Autodesk Inventor part; units mm, degrees
ref_plane "YZ Plane" through (0, 0, 0) normal (1, 0, 0) x (0, 1, 0)
ref_plane "XZ Plane" through (0, 0, 0) normal (0, 1, 0) x (-1, 0, 0)
ref_plane "XY Plane" through (0, 0, 0) normal (0, 0, 1) x (1, 0, 0)
sketch "Sketch1" plane through (0, 0, 0) normal (0, 0, 1) x (1, 0, 0)
  circle A0 centre (0, 0) radius 37.465
  dimension "d0" = 74.93
extrude "Extrusion1" add sketch "Sketch1" along normal blind 2.54
sketch "Sketch3" plane through (0, 0, 0) normal (0, 0, -1) x (-1, 0, 0)
  circle A0 centre (0, 0) radius 4.191
  circle A1 centre (0, 0) radius 7.9375
  circle A2 centre (0, 0) radius 2.3813
  dimension "d4" = 8.382
  dimension "d5" = 15.875
  dimension "d6" = 4.7625
extrude "Extrusion3" cut sketch "Sketch3" against normal through all contours A0 | A2
extrude "Extrusion4" add sketch "Sketch3" along normal blind 5.08 contours A1
sketch "Sketch4" plane through (0, 0, 2.54) normal (0, 0, 1) x (1, 0, 0)
  line L0 (0, 0) -> (0, 30.48)
  circle A0 centre (0, 30.48) radius 1.905
  circle A1 centre (-26.3965, 15.24) radius 1.905
  circle A2 centre (-26.3965, -15.24) radius 1.905
  circle A3 centre (0, -30.48) radius 1.905
  circle A4 centre (26.3965, -15.24) radius 1.905
  circle A5 centre (26.3965, 15.24) radius 1.905
  dimension "d13" = 30.48
  dimension "d14" = 3.81
  dimension "d17" = 360
extrude "Extrusion5" cut sketch "Sketch4" against normal blind 25.4
sketch "Sketch6" plane through (0, 0, 2.54) normal (0, 0, 1) x (1, 0, 0)
  circle A0 centre (0, 0) radius 3.556
  circle A1 centre (0, 0) radius 4.191
  dimension "d21" = 7.112
extrude "Extrusion6" add sketch "Sketch6" against normal blind 1.27
chamfer "Chamfer1" distance 1.27 angle 45 6 edges at (-28.3015, -15.24, 2.54) (-28.3015, 15.24, 2.54) (-1.905, 30.48, 2.54) (-1.905, -30.48, 2.54) (24.4915, -15.24, 2.54) (24.4915, 15.24, 2.54)
sketch "Sketch7" plane through (0, 0, 2.54) normal (0, 0, 1) x (1, 0, 0)
  circle A0 centre (0, 19.05) radius 3.175
  point P0 (0, 0)
  dimension "d27" = 6.35
  dimension "d28" = 19.05
extrude "Extrusion7" cut sketch "Sketch7" against normal through all
fillet "Fillet1" radius 1.27 1 edges at (7.9375, 0, 0)
properties part number "SpoolEndFrontSide"
Model file for the job. Use its own axes, mm. A direction names the side the tool comes from. Give positions to 0.01 mm unless a question says otherwise; leave off trailing zeros. Order: outer loops, then holes, each group sorted by start corner. A loop starts at its lowest first (then second) coordinate and runs counter-clockwise, first axis right, second up.
1) Saw through at B-B, the plane y = -15.24. Write the cut outline in (x, z).
2) Saw through at A-A, the plane x = 0. Count the separate pieces of the cut face and the enclosed holes in it, then the cut area to 3 significant figures.
3) Wall check: probe 1 along Y at (x, z) = (0, 1.7) (3 decimals); probe 2 along Z at (x, y) = (-23, -6.5); probe 3 along Y at (x, z) = (-23, 2). Give the ranges that are in metal, low to high.
4) Mould opens along Y. For faces 3 (the cylindrical face through (-26.81, 13.38, 0.64)), 4 (the flat face through (8, -8, 0)), 5 (the cylindrical face through (-29.73, 22.8, 1.25)), 6 (the cylindrical face through (-0.69, 15.95, 1.29)) say: +Y half, -Y half, draft (parallel to the pull), parting line (faces both ways), or undercut.
5) 3-axis set-ups, long thin cutter, end or side, ignore diameter. For faces 1 (the cylindrical face through (-3.997, -1.259, -1.861)), 2 (the cylindrical face through (25.98, 13.38, 0.64)): which of +Z, -Z, +X, -X, +Y, -Y reach the whole face in a straight line?
6) Saw through at D-D, the plane z = -3.25. Write the cut outline in (x, y) (1 decimal), then the cut area to 3 significant figures.
7) Saw through at C-C, the plane y = 30.48. Write the cut outline in (x, z) (3 decimals), then the cut area to 3 significant figures.
8) Pin check, flat tips, straight feed: pin 1 (4 mm diameter, centred on x = -7, z = 1.5, fed in from -Y); pin 2 (5 mm diameter, centred on x = 26.4, y = 15.24, fed in from -Z); pin 3 (5 mm diameter, centred on x = -26.4, y = -15.24, fed in from +Z). Stop position of each tip, or through.
Computed:
1. outline: (-34.23, 0) - (-28.3, 0) - (-28.3, 1.27) - (-29.57, 2.54) - (-34.23, 2.54) - close; (-24.49, 0) - (24.49, 0) - (24.49, 1.27) - (23.22, 2.54) - (-23.22, 2.54) - (-24.49, 1.27) - close; (28.3, 0) - (34.23, 0) - (34.23, 2.54) - (29.57, 2.54) - (28.3, 1.27) - close
2. separate pieces: 5
2. enclosed holes: 0
2. area: 171 mm2
3. probe 1: y = -37.465 to -32.815, -28.145 to -3.556, 3.556 to 15.875, 22.225 to 28.145, 32.815 to 37.465
3. probe 2: z = 0 to 2.54
3. probe 3: y = -29.57 to 29.57
4. face 3: undercut
4. face 4: draft
4. face 5: parting line
4. face 6: undercut
5. face 1: -Z
5. face 2: +Z, -Z
6. outline: circle Ø15.9 at (0, 0); hole circle Ø8.4 at (0, 0)
6. area: 143 mm2
7. outline: (-21.785, 0) - (-1.905, 0) - (-1.905, 1.27) - (-3.175, 2.54) - (-21.785, 2.54) - close; (1.905, 0) - (21.785, 0) - (21.785, 2.54) - (3.175, 2.54) - (1.905, 1.27) - close
7. area: 99.4 mm2
8. pin 1: stops at y = -37.13
8. pin 2: stops at z = 0
8. pin 3: stops at z = 1.87
